Could you check a few things on this model? Use its own coordinates, in mm. Face numbers are marked on the shaded views. Coordinates: 2 decimals unless noted, no trailing zeros. Order: outer loops, then holes, each group sorted by start corner. A loop starts at its lowest first (then second) coordinate and runs counter-clockwise, first axis right, second up. Notation, with made-up numbers: (37, -11) -> (79, -11) arc R29 cw to (79, 13) -> close; hole circle Ø6 at (-40, 4.25). An arc over 180 degrees is marked (long way). Use a Markdown table: item, result. Add a question column.
1) Thinking about a two-plate mould opening in Z: for the marked faces 1, 2 and 3, which applies, +Z half, -Z half, draft (parallel to the pull), parting line (faces both ways), or undercut?
2) If we section it at B-B (x = 21): Write out the boundary of the cut face in (y, z), plus the area to 3 significant figures.
3) If we section it at C-C (y = 1.75): Give the number of separate pieces and of enclosed holes in the cut face, plus the area to 3 significant figures.
4) If we section it at A-A (z = -16): Write out the boundary of the cut face in (x, y).
5) If I drill on L1, parallel to Z at x = 40, y = 4.75; L2, parallel to Z at x = 21, y = 7.6; L3, parallel to X at y = 3, z = 13.5, over which ranges is the centre line in solid material (lowest first)? Write a range as [from, to].
6) Will these pins go through, and if not, where does the flat tip stop? pin 1 Ø1.8 at (x, z) = (-40, 30) entering from +Y; pin 2 Ø2.5 at (x, z) = (22.5, 14.5) entering from -Y.
7) If we section it at D-D (z = -30): Write out the boundary of the cut face in (x, y), plus the area to 3 significant figures.
Solid Edge part; units mm, degrees
sketch "Sketch1" plane through (0, 0, 0) normal (0, -1, 0) x (1, 0, 0)
  line L0 (-45, -40) -> (45, -40)
  line L1 (45, -40) -> (45, 40)
  line L2 (45, 40) -> (-45, 40)
  line L3 (-45, 40) -> (-45, -40)
  dimension "D1" = 45
  dimension "D2" = 45
extrude "Protrusion1" add sketch "Sketch1" against normal blind 10
sketch "Sketch2" plane through (0, 0, 0) normal (0, -1, 0) x (1, 0, 0)
  circle A0 centre (-40, 30) radius 1
  circle A1 centre (-40, -30) radius 1
  circle A2 centre (40, -30) radius 1
  circle A3 centre (40, 30) radius 1
  dimension "D1" = 40
  dimension "D2" = 40
extrude "Cutout1" cut sketch "Sketch2" against normal through all
sketch "Sketch3" plane through (0, 0, 0) normal (0, -1, 0) x (1, 0, 0)
  circle A0 centre (-21, 16) radius 4
  circle A1 centre (-21, -16) radius 4
  circle A2 centre (21, -16) radius 4
  circle A3 centre (21, 16) radius 4
extrude "Extrusionsausschnitt_2" cut sketch "Sketch3" against normal blind 5
sketch "Sketch4" plane through (0, 0, 0) normal (0, -1, 0) x (1, 0, 0)
  circle A0 centre (-21, 16) radius 2
  circle A1 centre (-21, -16) radius 2
  circle A2 centre (21, -16) radius 2
  circle A3 centre (21, 16) radius 2
extrude "Cutout2" cut sketch "Sketch4" against normal through all
fillet "Verrundung_1" radius 4 4 edges at (-45, 5, 40) (45, 5, 40) (45, 5, -40) (-45, 5, -40)
properties material "Nylon, allgemein"
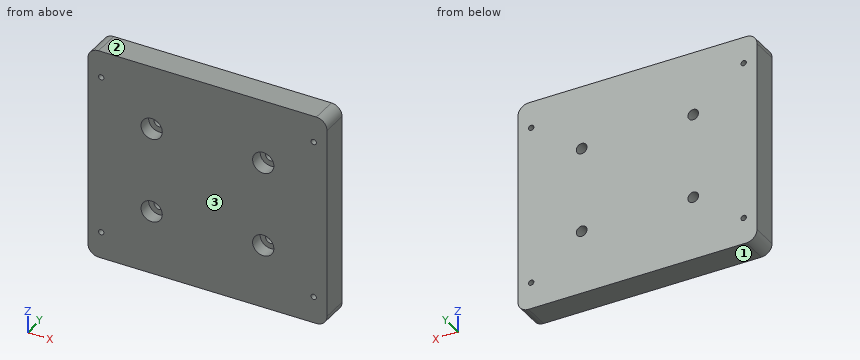
Answer sheet:
| question | item | result |
|---|---|---|
| 1 | face 1 | -Z half |
| 1 | face 2 | +Z half |
| 1 | face 3 | draft |
| 2 | outline | (0, -40) -> (10, -40) -> (10, -18) -> (5, -18) -> (5, -20) -> (0, -20) -> close; (0, -12) -> (5, -12) -> (5, -14) -> (10, -14) -> (10, 14) -> (5, 14) -> (5, 12) -> (0, 12) -> close; (0, 20) -> (5, 20) -> (5, 18) -> (10, 18) -> (10, 40) -> (0, 40) -> close |
| 2 | area | 680 mm2 |
| 3 | separate pieces | 1 |
| 3 | enclosed holes | 8 |
| 3 | area | 6,970 mm2 |
| 4 | outline | (-45, 0) -> (-25, 0) -> (-25, 5) -> (-23, 5) -> (-23, 10) -> (-45, 10) -> close; (-19, 5) -> (-17, 5) -> (-17, 0) -> (17, 0) -> (17, 5) -> (19, 5) -> (19, 10) -> (-19, 10) -> close; (23, 5) -> (25, 5) -> (25, 0) -> (45, 0) -> (45, 10) -> (23, 10) -> close |
| 5 | L1 | [-40, -31], [-29, 29], [31, 40] |
| 5 | L2 | [-40, -18], [-14, 14], [18, 40] |
| 5 | L3 | [-45, -24.12], [-17.88, 17.88], [24.12, 45] |
| 6 | pin 1 | through |
| 6 | pin 2 | y = 5 |
| 7 | outline | (-45, 0) -> (-41, 0) -> (-41, 10) -> (-45, 10) -> close; (-39, 0) -> (39, 0) -> (39, 10) -> (-39, 10) -> close; (41, 0) -> (45, 0) -> (45, 10) -> (41, 10) -> close |
| 7 | area | 860 mm2 |
